The model under review builds one solid part; all positions refer to its coordinate system, in mm. A direction names the side the tool comes from. Give positions to 0.01 mm unless a question says otherwise; leave off trailing zeros. Loops run counter-clockwise (first coordinate to the right, second up) from the corner with the lowest first, then second, coordinate; pieces in that order, holes last. Notation, with made-up numbers: M 38,21.25 L 88,21.25 A9 cw 88,36.25 Z; hole C -4,-4.75 d1. An arc over 180 degrees is marked long. One line per item, written item: value. Start each with the question number.
Q1. For faces 1 (the face through (11.86, -3, -87)), 2 (the face through (6, -3, -126.336)), 3 (the face through (4.663, -3.131, -33.465)), list the 3-axis set-ups (+Z, -Z, +X, -X, +Y, -Y) from which the entire face can be reached by the end or side of a thin tool; tool diameter is ignored.
Q2. We need section A-A on y = -1. Write out the cut boundary in (x, z).
Q3. To check wall thickness, follow line 1 along X through (y, z) = (-3.5, -86.5); line 2 along X through (y, z) = (-3.5, -12); line 3 along Z through (x, y) = (31, -4.75). State the ranges of each line that lie inside material, in increasing order. Write a range as from..to.
Q4. Mouldability with a two-part tool opening along Z and no side actions: class faces 4 (the face through (0, -3, -82)), 5 (the face through (72, -3, 21.803)), 6 (the face through (7.8, -3.13, -27.34)) as released by +Z, released by -Z, zero draft, split by the parting line, or undercut.
Q5. For pin 1 (1.5 mm diameter, centred on x = 33, y = -3, fed in from -Z); pin 2 (2 mm diameter, centred on x = 57, y = -2.5, fed in from -Z); pin 3 (3 mm diameter, centred on y = -3, z = -81, fed in from +X), all flat-tipped, find the tip position at first contact; note any pin that passes through.
Q6. We need section B-B on z = -109.5. Write out the cut boundary in (x, y), plus the area to 3 significant figures.
Q7. We need section C-C on x = 33. Write out the cut boundary in (y, z), plus the area to 3 significant figures.
```python
from build123d import *

# Parameters (mm, degrees)
F1_DEPTH = 6.35


with BuildPart() as f1:
    # F0 (on Front) → F1 (new body)
    with BuildSketch(Plane.XZ):
        with BuildLine():
            Line((75.361562, 21.802573), (68.159193, 21.802573))
            ThreePointArc((68.159193, 21.802573), (67.643768, 21.659507), (67.275821, 21.271246))
            ThreePointArc((67.275821, 21.271246), (39.236961, -8.061658), (0, -18.408534))
            Line((0, -18.408534), (0, -26.264148))
            Line((0, -26.264148), (6.028164, -26.264148))
            ThreePointArc((6.028164, -26.264148), (7.814478, -27.364658), (7.634936, -29.455065))
            Line((7.634936, -29.455065), (1.606772, -37.588195))
            ThreePointArc((1.606772, -37.588195), (0.89949, -38.183592), (0, -38.397278))
            Line((0, -38.397278), (0, -126.335785))
            Line((0, -126.335785), (11.859682, -126.335785))
            Line((11.859682, -126.335785), (11.859682, -46.803811))
            ThreePointArc((11.859682, -46.803811), (12.232361, -44.909636), (13.294841, -43.29783))
            Line((13.294841, -43.29783), (36.590743, -19.610819))
            ThreePointArc((36.590743, -19.610819), (37.801559, -18.56257), (39.164187, -17.721058))
            ThreePointArc((39.164187, -17.721058), (60.841409, -1.721337), (76.263449, 20.370601))
            ThreePointArc((76.263449, 20.370601), (76.207722, 21.335503), (75.361562, 21.802573))
        make_face()
    extrude(amount=F1_DEPTH)


solid = f1.part
```
Solved:
1. face 1: -Z, +X, +Y, -Y
1. face 2: -Z, +X, -X, +Y, -Y
1. face 3: -X, +Y, -Y
2. outline: M 0,-126.34 L 11.86,-126.34 L 11.86,-46.8 A5 cw 13.29,-43.3 L 36.59,-19.61 A10 cw 39.16,-17.72 A83.13 ccw 76.26,20.37 A1 ccw 75.36,21.8 L 68.16,21.8 A1 ccw 67.28,21.27 A74.7 cw 0,-18.41 L 0,-26.26 L 6.03,-26.26 A2 cw 7.63,-29.46 L 1.61,-37.59 A2 cw 0,-38.4 Z
3. line 1: 0..11.86
3. line 2: 31.58..48.71
3. line 3: -25.3..-12.26
4. face 4: zero draft
4. face 5: released by +Z
4. face 6: undercut
5. pin 1: z = -24.02
5. pin 2: z = -6.31
5. pin 3: x = 11.86
6. outline: M 0,-6.35 L 11.86,-6.35 L 11.86,0 L 0,0 Z
6. area: 75.3 mm2
7. outline: M -6.35,-23.26 L 0,-23.26 L 0,-11.35 L -6.35,-11.35 Z
7. area: 75.6 mm2
